from build123d import *

# Parameters (mm, degrees)
SALIENTE_EXTRUIR1_DEPTH = 15
CROQUIS2_OUTSIDE_W      = 78.456
CROQUIS2_OUTSIDE_H      = 73.814
CROQUIS2_OUTSIDE_R      = 16
CORTAR_EXTRUIR1_DEPTH   = 15
CORTAR_EXTRUIR1_TAPER   = 47
CROQUIS3_OUTSIDE_W      = 78.456
CROQUIS3_OUTSIDE_H      = 73.814
CROQUIS3_OUTSIDE_R      = 15
CORTAR_EXTRUIR2_DEPTH   = 15
CORTAR_EXTRUIR2_TAPER   = 47
CROQUIS4_R              = 8.25
CORTAR_EXTRUIR3_DEPTH   = 15
REDONDEO1_R             = 1


with BuildPart() as part:
    # Croquis1 → Saliente-Extruir1 (new body)
    with BuildSketch(Plane(origin=(0, 0, 0), x_dir=(1, 0, 0), z_dir=(0, 1, 0))):
        Polygon((-8.660254038, -15), (8.660254038, -15), (17.320508076, 0), (8.660254038, 15), (-8.660254038, 15), (-17.320508076, 0), align=None)
    extrude(amount=-SALIENTE_EXTRUIR1_DEPTH)

    # Croquis2 outside → Cortar-Extruir1 (cut)
    with BuildSketch(Plane(origin=(0, 0, 0), x_dir=(1, 0, 0), z_dir=(0, 1, 0))):
        Rectangle(CROQUIS2_OUTSIDE_W, CROQUIS2_OUTSIDE_H)
        Circle(CROQUIS2_OUTSIDE_R, mode=Mode.SUBTRACT)
    extrude(amount=-CORTAR_EXTRUIR1_DEPTH, taper=CORTAR_EXTRUIR1_TAPER, mode=Mode.SUBTRACT)

    # Croquis3 outside → Cortar-Extruir2 (cut)
    with BuildSketch(Plane.XZ.offset(15)):
        Rectangle(CROQUIS3_OUTSIDE_W, CROQUIS3_OUTSIDE_H)
        Circle(CROQUIS3_OUTSIDE_R, mode=Mode.SUBTRACT)
    extrude(amount=-CORTAR_EXTRUIR2_DEPTH, taper=CORTAR_EXTRUIR2_TAPER, mode=Mode.SUBTRACT)

    # Croquis4 → Cortar-Extruir3 (cut)
    with BuildSketch(Plane(origin=(0, 0, 0), x_dir=(1, 0, 0), z_dir=(0, 1, 0))):
        Circle(CROQUIS4_R)
    extrude(amount=-CORTAR_EXTRUIR3_DEPTH, mode=Mode.SUBTRACT)

    # Redondeo1
    redondeo1_edges = [part.edges().sort_by_distance(p)[0] for p in [
        (-8.25, -15, 0),
        (-8.25, 0, 0),
    ]]
    fillet(redondeo1_edges, radius=REDONDEO1_R)


solid = part.part
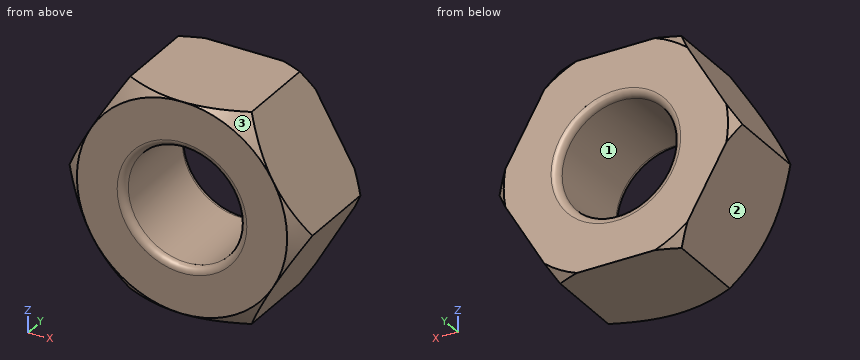
Here's how the part is built. I have some questions about the finished solid (model axes, mm). Face numbers are marked on the shaded views. Give positions to 0.01 mm unless a question says otherwise; leave off trailing zeros. Order: outer loops, then holes, each group sorted by start corner. A loop starts at its lowest first (then second) coordinate and runs counter-clockwise, first axis right, second up. Notation, with made-up numbers: (-6.75, 69.5) -> (46.25, 69.5) arc R30 cw to (46.25, 107.5) -> close; hole circle Ø8 at (-33, -20.75). An arc over 180 degrees is marked (long way). One line per item, written item: value. Start each with the question number.
1. We'd pull the mould along Z, two halves only. Please class the marked faces 1, 2 and 3: released by +Z, released by -Z, zero draft, split by the parting line, or undercut.
2. I need wall thicknesses on probe 1 along Z at (x, y) = (0, -6.75); probe 2 along X at (y, z) = (-9.25, 0); probe 3 along Z at (x, y) = (-6.5, -11). Which ranges of each line are inside material? Lowest first, please. Write a range as from..to.
3. Will these pins go through, and if not, where does the flat tip stop? pin 1 Ø1 at (y, z) = (-5, 10) entering from -X; pin 2 Ø5 at (y, z) = (-10.5, 11.5) entering from -X; pin 3 Ø8 at (x, z) = (-3.5, -1) entering from +Y.
4. Imagine slicing it at A-A, the plane y = -7.5. List the corners of the cut face in (x, z) for me.
Values follow:
1. face 1: undercut
1. face 2: released by -Z
1. face 3: released by +Z
2. probe 1: z = -15..-8.25, 8.25..15
2. probe 2: x = -17.32..-8.25, 8.25..17.32
2. probe 3: z = -15..-5.08, 5.08..15
3. pin 1: stops at x = -11.84
3. pin 2: stops at x = -12.12
3. pin 3: passes through
4. outline: (-17.32, 0) -> (-8.66, -15) -> (8.66, -15) -> (17.32, 0) -> (8.66, 15) -> (-8.66, 15) -> close; hole circle Ø16.5 at (0, 0)
